from build123d import *

# Parameters (mm, degrees)
SKETCH1_R           = 2.5
SKETCH1_R_2         = 6.35
BOSS_EXTRUDE1_DEPTH = 6
SKETCH2_R           = 9
SKETCH2_R_2         = 6.35
BOSS_EXTRUDE2_DEPTH = 51
FILLET1_R           = 3
CUT_EXTRUDE1_START  = -45
CUT_EXTRUDE1_DEPTH  = 45
FILLET2_R           = 0.5


with BuildPart() as part:
    # Sketch1 → Boss-Extrude1 (new body)
    with BuildSketch(Plane.XY):
        with BuildLine():
            ThreePointArc((17.324446131, 21.356815452), (0, 27.5), (-17.324446131, 21.356815452))
            ThreePointArc((-17.324446131, 21.356815452), (-15.155444566, 8.75), (-27.157767791, 4.325002729))
            ThreePointArc((-27.157767791, 4.325002729), (-23.815698604, -13.75), (-9.83332166, -25.681818182))
            ThreePointArc((-9.83332166, -25.681818182), (0, -17.5), (9.83332166, -25.681818182))
            ThreePointArc((9.83332166, -25.681818182), (23.815698604, -13.75), (27.157767791, 4.325002729))
            ThreePointArc((27.157767791, 4.325002729), (15.155444566, 8.75), (17.324446131, 21.356815452))
        make_face()
        with Locations((0, 23.75)):
            Circle(SKETCH1_R, mode=Mode.SUBTRACT)
        with Locations((-20.56810334, -11.875)):
            Circle(SKETCH1_R, mode=Mode.SUBTRACT)
        with Locations((20.56810334, -11.875)):
            Circle(SKETCH1_R, mode=Mode.SUBTRACT)
        Circle(SKETCH1_R_2, mode=Mode.SUBTRACT)
    extrude(amount=BOSS_EXTRUDE1_DEPTH)

    # Sketch2 → Boss-Extrude2 (add)
    with BuildSketch(Plane.XY.offset(6)):
        Circle(SKETCH2_R)
        Circle(SKETCH2_R_2, mode=Mode.SUBTRACT)
    extrude(amount=BOSS_EXTRUDE2_DEPTH)

    # Fillet1
    fillet1_edges = [part.edges().sort_by_distance(p)[0] for p in [
        (27.157767791, 4.325002729, 3),
        (9.83332166, -25.681818182, 3),
        (-9.83332166, -25.681818182, 3),
        (-27.157767791, 4.325002729, 3),
        (-17.324446131, 21.356815452, 3),
        (17.324446131, 21.356815452, 3),
    ]]
    fillet(fillet1_edges, radius=FILLET1_R)

    # Sketch3 → Cut-Extrude1 (cut)
    with BuildSketch(Plane.XY.offset(57).offset(CUT_EXTRUDE1_START)):
        with BuildLine():
            Line((-1.5, 6.170291727), (-1.5, 7.170291727))
            Line((-1.5, 7.170291727), (1.5, 7.170291727))
            Line((1.5, 7.170291727), (1.5, 6.170291727))
            ThreePointArc((1.5, 6.170291727), (0, 6.35), (-1.5, 6.170291727))
        make_face()
    extrude(amount=CUT_EXTRUDE1_DEPTH, mode=Mode.SUBTRACT)

    # Fillet2
    fillet2_edges = [part.edges().sort_by_distance(p)[0] for p in [
        (-9, 0, 6),
    ]]
    fillet(fillet2_edges, radius=FILLET2_R)


solid = part.part
The listing builds one solid part. Answer for the finished solid, in the listing's coordinates (mm). A direction names the side the tool comes from. Give positions to 0.01 mm unless a question says otherwise; leave off trailing zeros. Loops run counter-clockwise (first coordinate to the right, second up) from the corner with the lowest first, then second, coordinate; pieces in that order, holes last. Notation, with made-up numbers: (-13, -18.75) - (31, -18.75) arc R13 cw to (31, 1.25) - close; hole circle Ø5 at (-17, 58). An arc over 180 degrees is marked (long way). Use one line per item in the form item = value.
1. Which of the six approach directions +Z, -Z, +X, -X, +Y, -Y give full straight-line access (tool end or side, diameter ignored) to faces 1 (the face through (0, 7.17, 34)), 2 (the face through (4, -6, 57))?
Calculated:
face_1 = +Z
face_2 = +Z, +X, -X, +Y, -Y
2. Section C-C on z = 33.5 is taken. Give the vertices of the cut face in (x, y).
Calculated:
outline = circle Ø18 at (0, 0); hole (-1.5, 6.17) arc R6.35 ccw (long way) to (1.5, 6.17) - (1.5, 7.17) - (-1.5, 7.17) - close
3. Section B-B on y = 0 is taken. Give the vertices of the cut face in (x, z).
Calculated:
outline = (-27.5, 0) - (-6.35, 0) - (-6.35, 57) - (-9, 57) - (-9, 6.5) arc R0.5 cw to (-9.5, 6) - (-27.5, 6) - close; (6.35, 0) - (27.5, 0) - (27.5, 6) - (9.5, 6) arc R0.5 cw to (9, 6.5) - (9, 57) - (6.35, 57) - close
4. Find the intervals of material crossed by line 1 along Y through (x, z) = (0, 40.5); line 2 along Z through (x, y) = (5.5, 13); line 3 along X through (y, z) = (3, 24), in increasing order. Write a range as [from, to].
Calculated:
line_1 = [-9, -6.35], [7.17, 9]
line_2 = [0, 6]
line_3 = [-8.49, -5.6], [5.6, 8.49]
5. Section D-D on z = 5 is taken. Count the separate pieces of the cut face and the enclosed holes in it, then the cut area to 3 significant figures.
Calculated:
separate_pieces = 1
enclosed_holes = 4
area = 1,740 mm^2
6. Section A-A on x = 0 is taken. Give the vertices of the cut face in (y, z), then the cut area to 3 significant figures.
Calculated:
outline = (-17.5, 0) - (-6.35, 0) - (-6.35, 57) - (-9, 57) - (-9, 6.5) arc R0.5 cw to (-9.5, 6) - (-17.5, 6) - close; (6.35, 0) - (21.25, 0) - (21.25, 6) - (9.5, 6) arc R0.5 cw to (9, 6.5) - (9, 57) - (7.17, 57) - (7.17, 12) - (6.35, 12) - close; (26.25, 0) - (27.5, 0) - (27.5, 6) - (26.25, 6) - close
area = 397 mm^2
7. The mould has two halves that part along Y. Classify faces 3 (the face through (0, -10, 6)), 4 (the face through (-0.2, -17.5, 3)), 5 (the face through (-1.172, 8.923, 31.396)), 6 (the face through (21.722, -14.093, 2.958)): pulls with the +Y half, pulls with the -Y half, needs draft (parallel to the pull), parting line crosses it, or undercut.
Calculated:
face_3 = needs draft
face_4 = pulls with the -Y half
face_5 = parting line crosses it
face_6 = undercut
8. Given pin 1 Ø0.8 at (y, z) = (6.5, 40) entering from -X; pin 2 Ø6 at (x, y) = (20.57, -11.88) entering from +Z; pin 3 Ø3.5 at (x, z) = (0, 43.5) entering from -Y, each flat-ended and moving along its own axis, determine where each tip first touches the part or whether it passes through.
Calculated:
pin_1 = -6.62
pin_2 = 6
pin_3 = -9
